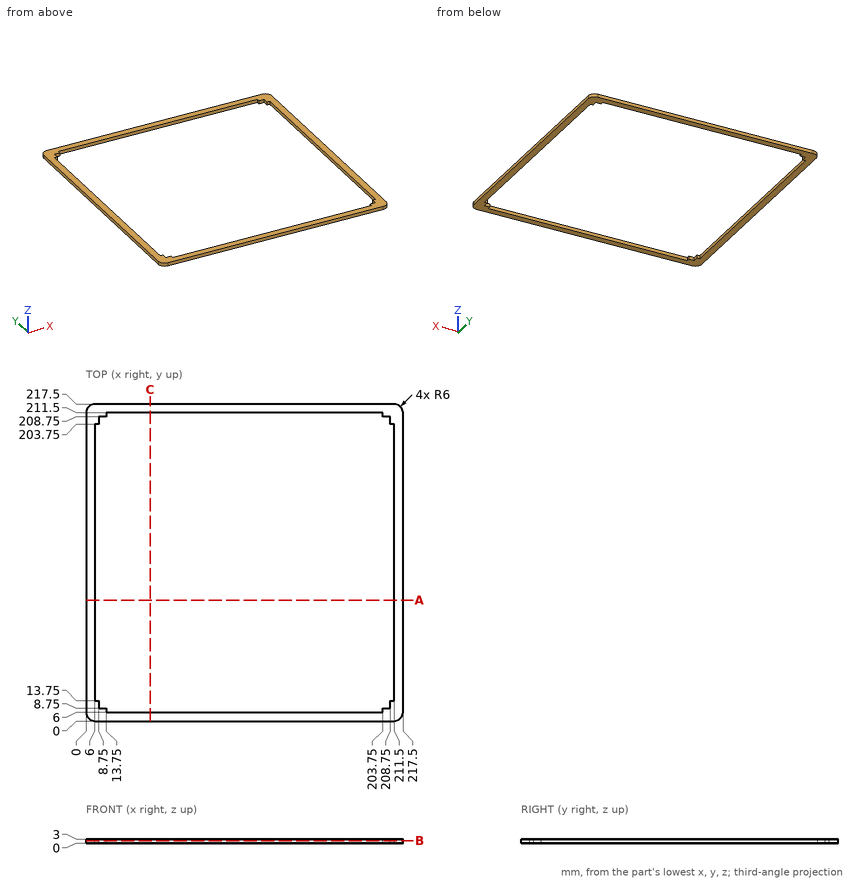
Study the drawing (mm; zero at the part's minimum x, y, z) and answer. Round coordinates to 2 decimals unless told otherwise and drop trailing zeros. Order: outer loops, then holes, each group sorted by start corner. A loop starts at its lowest first (then second) coordinate and runs counter-clockwise, first axis right, second up. Notation, with made-up numbers: (42.25, 72) - (84.25, 72) arc R14 ccw to (84.25, 99) - close; hole circle Ø11 at (78.25, -15.75). An arc over 180 degrees is marked (long way). Use one line per item in the form item = value. Start each with the question number.
(1) The part is cut by section A-A (y = 83). Give the vertices of the cut face in (x, z), then the cut area to 3 significant figures.
(2) The part is cut by section B-B (z = 1.95). Give the vertices of the cut face in (x, y).
(3) Find the intervals of material crossed by line 1 along X through (y, z) = (26, 1.75); line 2 along X through (y, z) = (10, 1.15), in increasing order. Write a range as from..to.
Checked values:
q1.outline = (0, 0) - (6, 0) - (6, 3) - (0, 3) - close; (211.5, 0) - (217.5, 0) - (217.5, 3) - (211.5, 3) - close
q1.area = 36.0 mm^2
q2.outline = (0, 6) arc R6 ccw to (6, 0) - (211.5, 0) arc R6 ccw to (217.5, 6) - (217.5, 211.5) arc R6 ccw to (211.5, 217.5) - (6, 217.5) arc R6 ccw to (0, 211.5) - close; hole (6, 13.75) - (8.75, 13.75) - (8.75, 8.75) - (13.75, 8.75) - (13.75, 6) - (203.75, 6) - (203.75, 8.75) - (208.75, 8.75) - (208.75, 13.75) - (211.5, 13.75) - (211.5, 203.75) - (208.75, 203.75) - (208.75, 208.75) - (203.75, 208.75) - (203.75, 211.5) - (13.75, 211.5) - (13.75, 208.75) - (8.75, 208.75) - (8.75, 203.75) - (6, 203.75) - close
q3.line_1 = 0..6, 211.5..217.5
q3.line_2 = 0..8.75, 208.75..217.5
